Drawing for the job (mm, zero at the part's lowest x, y, z). A direction names the side the tool comes from. Give positions to 0.01 mm unless a question says otherwise; leave off trailing zeros. Order: outer loops, then holes, each group sorted by start corner. A loop starts at its lowest first (then second) coordinate and runs counter-clockwise, first axis right, second up. Notation, with made-up numbers: (-22, 13) -> (32, 13) arc R28 ccw to (32, 33) -> close; hole circle Ø3 at (84, 53). An arc over 180 degrees is marked (long way). Use a Markdown table: item, result. Add a question column.
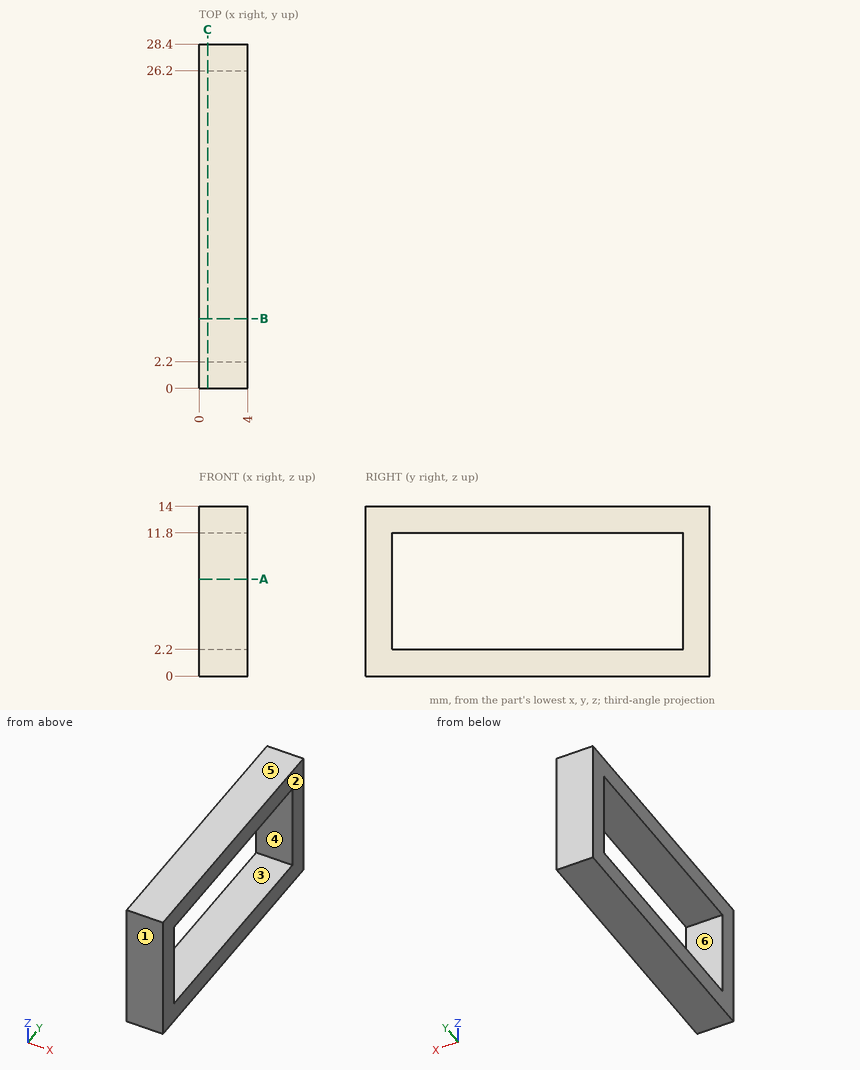
(1) Tool access for the marked faces 5 and 6: list every direction of +Z, -Z, +X, -X, +Y, -Y with a clear straight run to the whole face (end or side of a thin tool).
(2) Mould opens along Y. For the marked faces 1, 2, 3 and 4 say: released by +Y, released by -Y, zero draft, split by the parting line, or undercut.
(3) Wall check: probe 1 along Y at (x, z) = (0.65, 10); probe 2 along Z at (x, y) = (2.7, 3.5). Give the ranges that are in metal, low to high.
(4) Band-saw the part on A-A on z = 8. Give the cut face in (x, y), plus the area to 3 significant figures.
(5) Band-saw the part on C-C on x = 0.7. Give the cut face in (y, z), plus the area to 3 significant figures.
(6) Pin check, flat tip, straight feed: pin 1 Ø2 at (y, z) = (24, 10) entering from +X. Stop position of the tip, or through.
(7) Band-saw the part on B-B on y = 5.75. Give the cut face in (x, z).
Response:
| question | item | result |
|---|---|---|
| 1 | face 5 | +Z, +X, -X, +Y, -Y |
| 1 | face 6 | +X, -X |
| 2 | face 1 | released by -Y |
| 2 | face 2 | zero draft |
| 2 | face 3 | undercut |
| 2 | face 4 | undercut |
| 3 | probe 1 | y = 0 to 2.2, 26.2 to 28.4 |
| 3 | probe 2 | z = 0 to 2.2, 11.8 to 14 |
| 4 | outline | (0, 0) -> (4, 0) -> (4, 2.2) -> (0, 2.2) -> close; (0, 26.2) -> (4, 26.2) -> (4, 28.4) -> (0, 28.4) -> close |
| 4 | area | 17.6 mm² |
| 5 | outline | (0, 0) -> (28.4, 0) -> (28.4, 14) -> (0, 14) -> close; hole (2.2, 2.2) -> (26.2, 2.2) -> (26.2, 11.8) -> (2.2, 11.8) -> close |
| 5 | area | 167 mm² |
| 6 | pin 1 | passes through |
| 7 | outline | (0, 0) -> (4, 0) -> (4, 2.2) -> (0, 2.2) -> close; (0, 11.8) -> (4, 11.8) -> (4, 14) -> (0, 14) -> close |
